Autodesk Inventor part; units mm, degrees
ref_plane "Work Plane1" through (7.995, 0, 0) normal (1, 0, 0) x (0, 1, 0)
ref_plane "XZ Plane" through (0, 0, 0) normal (0, 1, 0) x (-1, 0, 0)
ref_plane "XY Plane" through (0, 0, 0) normal (0, 0, 1) x (1, 0, 0)
sketch "Sketch1" plane through (0, 0, 0) normal (0, 1, 0) x (-1, 0, 0)
  line L0 (24, 221.2) -> (24, -221.2)
  line L1 (-24, -220.2) -> (-24, 220.2)
  arc A0 (-23, 221.2) -> (-24, 220.2) centre (-23, 220.2) ccw
  arc A1 (-24, -220.2) -> (-23, -221.2) centre (-23, -220.2) ccw
  line L2 (0, 0) -> (-12.5, 0)
  line L3 (-23, 221.2) -> (24, 221.2)
  line L4 (-23, -221.2) -> (24, -221.2)
  point P0 (-24, -221.2)
  dimension "d0" = 442.4
  dimension "d1" = 48
  dimension "d2" = 1
  dimension "d3" = 1
  dimension "d58" = 221.2
extrude "Extrusion1" add sketch "Sketch1" along normal blind 1.6
ref_plane "Work Plane1" through (7.995, 0, 0) normal (1, 0, 0) x (0, 1, 0)
sketch "Sketch4" plane through (0, 1.6, 0) normal (0, 1, 0) x (1, 0, 0)
  line L0 (-24, -221.2) -> (23, -221.2)
  line L1 (23, -221.2) -> (15, -221.2)
  line L2 (11, -219.6) -> (23, -219.6)
  line L3 (23, -219.6) -> (23, -221.2)
  line L4 (23, -221.2) -> (11, -221.2)
  line L5 (11, -221.2) -> (11, -219.6)
  line L6 (23, -221.2) -> (22, -221.2)
  line L7 (24, -220.2) -> (24, 220.2)
  point P0 (0, 0)
  dimension "d46" = 8
  dimension "d48" = 12
  dimension "d57" = 1
extrude "Extrusion4" add sketch "Sketch4" along normal blind 6
sketch "Sketch5" plane through (-24, 0, 221.2) normal (0, 0, 1) x (1, 0, 0)
  line L0 (35, 1.6) -> (47, 1.6)
  line L1 (47, 1.6) -> (47, 7.6)
  line L2 (47, 7.6) -> (35, 7.6)
  line L3 (0, 1.6) -> (35, 1.6)
  circle A0 centre (40.9972, 4.6) radius 2
  line L4 (35, 1.6) -> (47, 7.6)
  line L5 (35, 7.6) -> (47, 1.6)
  point P0 (24, 0)
  dimension "d52" = 4
extrude "Extrusion5" cut sketch "Sketch5" against normal blind 6 contours L4 L5 A0 | A0 L5 L4 | L5 L4 A0 | A0 L4 L5
fillet "Fillet3" radius 2 2 edges at (23, 7.6, 220.4) (11, 7.6, 220.4)
mirror "Mirror5" about plane through (7.995, 0, 0) normal (1, 0, 0) of "Extrusion4", "Extrusion5", "Fillet3"
mirror "Mirror6" about plane through (0, 0, 0) normal (0, 0, 1) of "Extrusion4", "Extrusion5", "Fillet3", "Mirror5"
properties part number "Caja - Pared"
Work out the finished part from the listing and answer in its coordinate system (mm). Give positions to 0.01 mm unless a question says otherwise; leave off trailing zeros. Loops run counter-clockwise (first coordinate to the right, second up) from the corner with the lowest first, then second, coordinate; pieces in that order, holes last. Notation, with made-up numbers: (56.25, -9) - (83.25, -9) arc R29 ccw to (83.25, 13) - close; hole circle Ø5 at (-17, 71.25). An arc over 180 degrees is marked (long way). One line per question, with ' | ' between items.
(1) Straight lines are drawn through the part: probe 1 along X at (y, z) = (4.6, -220.05); probe 2 along Z at (x, y) = (19.5, 7.25); probe 3 along Y at (x, z) = (16.5, -180). For each, find the intervals that lie inside material, in ascending order.
Recorded:
probe 1: x = -7.01 to -3.01, 0.99 to 4.99, 11 to 15, 19 to 23 | probe 2: z = -221.2 to -219.6, 219.6 to 221.2 | probe 3: y = 0 to 1.6
(2) The mould has two halves that part along Z. Classify faces 1 (the face through (5, 1, -221.2)), 2 (the face through (0, 0, 3)), 3 (the face through (0, 1.6, 3)): +Z half, -Z half, draft (parallel to the pull), parting line (faces both ways), or undercut.
Recorded:
face 1: -Z half | face 2: draft | face 3: undercut
(3) The part is cut by section B-B (x = -17). Write down the section's boundary in (y, z), then the cut area to 3 significant figures.
Recorded:
outline: (0, -221.2) - (1.6, -221.2) - (1.6, 221.2) - (0, 221.2) - close | area: 708 mm²
(4) Each of these flat-tipped pins is pushed along its axis until it touches: pin 1 Ø0.5 at (y, z) = (3, 220.5) entering from -X; pin 2 Ø5 at (x, z) = (-11.5, 12) entering from +Y; pin 3 Ø0.5 at (y, z) = (4.5, 220) entering from +X. Where does it stop, or does it pass through?
Recorded:
pin 1: stops at x = -7.01 | pin 2: stops at y = 1.6 | pin 3: stops at x = 23
(5) The part is cut by section A-A (z = 166). Write down the section's boundary in (x, y), then the cut area to 3 significant figures.
Recorded:
outline: (-24, 0) - (24, 0) - (24, 1.6) - (-24, 1.6) - close | area: 76.8 mm²
